Geometry check sheet. Reference: drawing and pictorial views, mm from the part's lowest x, y, z. Give positions to 0.01 mm unless a question says otherwise; leave off trailing zeros. Write each loop counter-clockwise with the first axis right and the second up, starting at its lowest first coordinate (ties: lowest second). Pieces come first, ordered by that corner, then holes. Notation, with made-up numbers: M -38,72 L 20,72 A11 ccw 20,77 Z; hole C -29.75,26 d8. An arc over 180 degrees is marked long. Write item = value, one per line. Start each with the question number.
1) Cross-section at C-C, the plane z = 20.75. Record the cut outline in (x, y) (3 decimals).
2) Scan lines: line 1 along X through (y, z) = (1.1, 8.68); line 2 along X through (y, z) = (0.75, 10.25); line 3 along Z through (x, y) = (38, 0.55). Record each from-to range of solid material in increasing order. Write a range as [from, to].
3) Cross-section at B-B, the plane y = 1. Give the number of separate pieces and of enclosed holes in the cut face, plus the area to 3 significant figures.
4) Cross-section at D-D, the plane x = 28. Record the cut outline in (y, z) (3 decimals).
5) Mould release check, pull along Z, two halves, no side actions. Record for the marked faces 1, 2, 3 and 4: released by +Z, released by -Z, zero draft, split by the parting line, or undercut.
6) Cross-section at A-A, the plane x = 21.5. Record the cut outline in (y, z) (3 decimals).
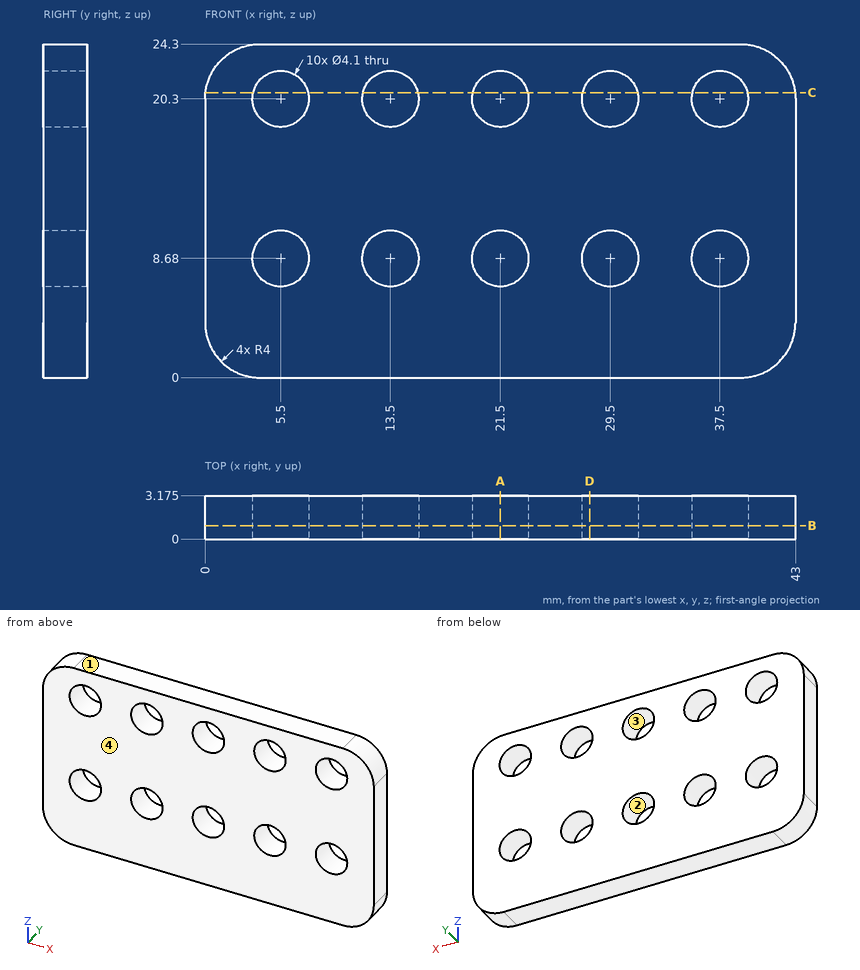
Reply:
q1.outline = M 0.025,0 L 3.5,0 L 3.5,3.175 L 0.025,3.175 Z; M 7.5,0 L 11.5,0 L 11.5,3.175 L 7.5,3.175 Z; M 15.5,0 L 19.5,0 L 19.5,3.175 L 15.5,3.175 Z; M 23.5,0 L 27.5,0 L 27.5,3.175 L 23.5,3.175 Z; M 31.5,0 L 35.5,0 L 35.5,3.175 L 31.5,3.175 Z; M 39.5,0 L 42.975,0 L 42.975,3.175 L 39.5,3.175 Z
q2.line_1 = [0, 3.45], [7.55, 11.45], [15.55, 19.45], [23.55, 27.45], [31.55, 35.45], [39.55, 43]
q2.line_2 = [0, 4.18], [6.82, 12.18], [14.82, 20.18], [22.82, 28.18], [30.82, 36.18], [38.82, 43]
q2.line_3 = [0, 6.69], [10.67, 18.31], [22.29, 24.3]
q3.separate_pieces = 1
q3.enclosed_holes = 10
q3.area = 899 mm2
q4.outline = M 0,0 L 3.175,0 L 3.175,7.283 L 0,7.283 Z; M 0,10.077 L 3.175,10.077 L 3.175,18.903 L 0,18.903 Z; M 0,21.697 L 3.175,21.697 L 3.175,24.3 L 0,24.3 Z
q5.face_1 = released by +Z
q5.face_2 = undercut
q5.face_3 = undercut
q5.face_4 = zero draft
q6.outline = M 0,0 L 3.175,0 L 3.175,6.63 L 0,6.63 Z; M 0,10.73 L 3.175,10.73 L 3.175,18.25 L 0,18.25 Z; M 0,22.35 L 3.175,22.35 L 3.175,24.3 L 0,24.3 Z
